from build123d import *

# Parameters (mm, degrees)
SKETCH1_W           = 27
SKETCH1_H           = 27
BOSS_EXTRUDE2_DEPTH = 75
SHELL1_T            = -1
SCALE1_SCALE        = 5


with BuildPart() as part:
    # Sketch1 → Boss-Extrude2 (new body)
    with BuildSketch(Plane(origin=(0, 0, 0), x_dir=(1, 0, 0), z_dir=(0, 1, 0))):
        Rectangle(SKETCH1_W, SKETCH1_H)
    extrude(amount=BOSS_EXTRUDE2_DEPTH)

    # Shell1
    shell1_openings = [part.faces().sort_by_distance(p)[0] for p in [
        (0, 75, 0),
    ]]
    offset(amount=SHELL1_T, openings=shell1_openings, kind=Kind.INTERSECTION)


with BuildPart() as part_1:
    # Scale1: scaled about (0, 0, 0)
    add(part.part.scale(SCALE1_SCALE))


solid = part_1.part
The listing builds one solid part. Answer for the finished solid, in the listing's coordinates (mm). A direction names the side the tool comes from. Coordinates: 2 decimals unless noted, no trailing zeros. Loops run counter-clockwise (first coordinate to the right, second up) from the corner with the lowest first, then second, coordinate; pieces in that order, holes last. Notation, with made-up numbers: (58, -33) -> (101, -33) arc R26 cw to (101, -11) -> close; hole circle Ø2 at (-29.75, -40). An arc over 180 degrees is marked (long way). Answer in a Markdown table with one row per item. Add a question column.
1. Determine the mould class of faces 1 (the flat face through (-1, 0, -1)), 2 (the flat face through (-1, 187, 62.5)), 3 (the flat face through (-67.5, 185, 1)) for opening direction X: +X half, -X half, draft (parallel to the pull), parting line (faces both ways), or undercut.
2. The part is cut by section C-C, the plane z = 34.5. Write down the section's boundary in (x, y).
3. For faces 4 (the flat face through (-62.5, 187, 1)), 5 (the flat face through (-1, 185, 67.5)), determine the directions among +Z, -Z, +X, -X, +Y, -Y from which every point of the face is accessible in a straight line to the end or side of a thin tool.
4. The part is cut by section A-A, the plane y = 83. Write down the section's boundary in (x, z), then the cut area to 3 significant figures.
5. A flat-ended cylindrical pin translates along its axis: P1, Ø1, axis at x = 24, z = -53, coming from the +Y side. Find the tip coordinate at first contact, or state that the pin passes through.
6. Consider line 1 (X direction, y = 199, z = 31.5); line 2 (Y direction, x = -38, z = -56.5). Determine where each line is inside the solid, lowest interval first. Write a range as [from, to].
7. The part is cut by section B-B, the plane x = 23.5. Write down the section's boundary in (y, z).
Answer below:
| question | item | result |
|---|---|---|
| 1 | face 1 | draft |
| 1 | face 2 | undercut |
| 1 | face 3 | -X half |
| 2 | outline | (-67.5, 0) -> (67.5, 0) -> (67.5, 375) -> (62.5, 375) -> (62.5, 5) -> (-62.5, 5) -> (-62.5, 375) -> (-67.5, 375) -> close |
| 3 | face 4 | +Y |
| 3 | face 5 | +Z, +X, -X, +Y, -Y |
| 4 | outline | (-67.5, -67.5) -> (67.5, -67.5) -> (67.5, 67.5) -> (-67.5, 67.5) -> close; hole (-62.5, -62.5) -> (62.5, -62.5) -> (62.5, 62.5) -> (-62.5, 62.5) -> close |
| 4 | area | 2,600 mm2 |
| 5 | P1 | y = 5 |
| 6 | line 1 | [-67.5, -62.5], [62.5, 67.5] |
| 6 | line 2 | [0, 5] |
| 7 | outline | (0, -67.5) -> (375, -67.5) -> (375, -62.5) -> (5, -62.5) -> (5, 62.5) -> (375, 62.5) -> (375, 67.5) -> (0, 67.5) -> close |
